For this review, take the finished solid that the model builds, in its own axes (mm). Coordinates: 2 decimals unless noted, no trailing zeros. Write each loop counter-clockwise with the first axis right and the second up, starting at its lowest first coordinate (ties: lowest second). Pieces come first, ordered by that corner, then holes. Notation, with made-up numbers: (2, 5.5) -> (21, 5.5) arc R23 cw to (21, 18.5) -> close; hole circle Ø7 at (77, -21). An arc over 180 degrees is marked (long way). Put each result on its own line as item: value. Start each with the question number.
Item 1: Consider section B-B on z = -168. Give the boundary of the cut face in (x, y) (3 decimals), and give its area (3 significant figures).
Item 2: Consider section A-A on y = 0.7. Give the boundary of the cut face in (x, z).
Item 3: Consider section C-C on x = 312.5. Give the boundary of the cut face in (y, z) (3 decimals).
Item 4: To check wall thickness, follow L1, parallel to Z at x = -130, y = 1.15; L2, parallel to X at y = 1.05, z = -150; L3, parallel to X at y = 2.15, z = -210. State the ranges of each line that lie inside material, in increasing order.
```python
from build123d import *

# Parameters (mm, degrees)
BOSS_EXTRUDE1_DEPTH = 3.175
CUT_EXTRUDE1_REACH  = 850.534


with BuildPart() as part:
    # Sketch1 → Boss-Extrude1 (new body)
    with BuildSketch(Plane(origin=(0, 0, 0), x_dir=(1, 0, 0), z_dir=(0, 1, 0))):
        with BuildLine():
            Line((-600, 0), (600, 0))
            ThreePointArc((600, 0), (0, 600), (-600, 0))
        make_face()
    extrude(amount=BOSS_EXTRUDE1_DEPTH)

    # Sketch2 → Cut-Extrude1 (cut, up to next)
    with BuildSketch(Plane(origin=(0, 3.175, 0), x_dir=(1, 0, 0), z_dir=(0, 1, 0)), mode=Mode.PRIVATE) as cut_extrude1_sk1:
        with BuildLine():
            Line((-130, 205), (-130, 210))
            Line((-130, 210), (-125, 210))
            ThreePointArc((-125, 210), (-133.535533906, 213.535533906), (-130, 205))
        make_face()
    cut_extrude1_tool1 = extrude(cut_extrude1_sk1.sketch, amount=-CUT_EXTRUDE1_REACH, mode=Mode.PRIVATE) & part.part
    # Sketch2 → Cut-Extrude1 (cut, up to next)
    with BuildSketch(Plane(origin=(0, 3.175, 0), x_dir=(1, 0, 0), z_dir=(0, 1, 0)), mode=Mode.PRIVATE) as cut_extrude1_sk2:
        with BuildLine():
            Line((-125, 210), (-130, 210))
            Line((-130, 210), (-130, 205))
            ThreePointArc((-130, 205), (-126.464466094, 206.464466094), (-125, 210))
        make_face()
    cut_extrude1_tool2 = extrude(cut_extrude1_sk2.sketch, amount=-CUT_EXTRUDE1_REACH, mode=Mode.PRIVATE) & part.part
    # Sketch2 → Cut-Extrude1 (cut, up to next)
    with BuildSketch(Plane(origin=(0, 3.175, 0), x_dir=(1, 0, 0), z_dir=(0, 1, 0)), mode=Mode.PRIVATE) as cut_extrude1_sk3:
        with BuildLine():
            Line((-130, 205), (-130, 210))
            Line((-130, 210), (-125, 210))
            ThreePointArc((-125, 210), (-133.535533906, 213.535533906), (-130, 205))
        make_face()
    cut_extrude1_tool3 = extrude(cut_extrude1_sk3.sketch, amount=-CUT_EXTRUDE1_REACH, mode=Mode.PRIVATE) & part.part
    # Sketch2 → Cut-Extrude1 (cut, up to next)
    with BuildSketch(Plane(origin=(0, 3.175, 0), x_dir=(1, 0, 0), z_dir=(0, 1, 0)), mode=Mode.PRIVATE) as cut_extrude1_sk4:
        with BuildLine():
            Line((-125, 210), (-130, 210))
            Line((-130, 210), (-130, 205))
            ThreePointArc((-130, 205), (-126.464466094, 206.464466094), (-125, 210))
        make_face()
    cut_extrude1_tool4 = extrude(cut_extrude1_sk4.sketch, amount=-CUT_EXTRUDE1_REACH, mode=Mode.PRIVATE) & part.part
    # Sketch2 → Cut-Extrude1 (cut, up to next)
    with BuildSketch(Plane(origin=(0, 3.175, 0), x_dir=(1, 0, 0), z_dir=(0, 1, 0)), mode=Mode.PRIVATE) as cut_extrude1_sk5:
        with BuildLine():
            ThreePointArc((-125, 150), (-126.464466094, 153.535533906), (-130, 155))
            Line((-130, 155), (-130, 150))
            Line((-130, 150), (-125, 150))
        make_face()
    cut_extrude1_tool5 = extrude(cut_extrude1_sk5.sketch, amount=-CUT_EXTRUDE1_REACH, mode=Mode.PRIVATE) & part.part
    # Sketch2 → Cut-Extrude1 (cut, up to next)
    with BuildSketch(Plane(origin=(0, 3.175, 0), x_dir=(1, 0, 0), z_dir=(0, 1, 0)), mode=Mode.PRIVATE) as cut_extrude1_sk6:
        with BuildLine():
            Line((-130, 150), (-130, 155))
            ThreePointArc((-130, 155), (-133.535533906, 146.464466094), (-125, 150))
            Line((-125, 150), (-130, 150))
        make_face()
    cut_extrude1_tool6 = extrude(cut_extrude1_sk6.sketch, amount=-CUT_EXTRUDE1_REACH, mode=Mode.PRIVATE) & part.part
    # Sketch2 → Cut-Extrude1 (cut, up to next)
    with BuildSketch(Plane(origin=(0, 3.175, 0), x_dir=(1, 0, 0), z_dir=(0, 1, 0)), mode=Mode.PRIVATE) as cut_extrude1_sk7:
        with BuildLine():
            ThreePointArc((-125, 150), (-126.464466094, 153.535533906), (-130, 155))
            Line((-130, 155), (-130, 150))
            Line((-130, 150), (-125, 150))
        make_face()
    cut_extrude1_tool7 = extrude(cut_extrude1_sk7.sketch, amount=-CUT_EXTRUDE1_REACH, mode=Mode.PRIVATE) & part.part
    # Sketch2 → Cut-Extrude1 (cut, up to next)
    with BuildSketch(Plane(origin=(0, 3.175, 0), x_dir=(1, 0, 0), z_dir=(0, 1, 0)), mode=Mode.PRIVATE) as cut_extrude1_sk8:
        with BuildLine():
            Line((-130, 150), (-130, 155))
            ThreePointArc((-130, 155), (-133.535533906, 146.464466094), (-125, 150))
            Line((-125, 150), (-130, 150))
        make_face()
    cut_extrude1_tool8 = extrude(cut_extrude1_sk8.sketch, amount=-CUT_EXTRUDE1_REACH, mode=Mode.PRIVATE) & part.part
    # Sketch2 → Cut-Extrude1 (cut, up to next)
    with BuildSketch(Plane(origin=(0, 3.175, 0), x_dir=(1, 0, 0), z_dir=(0, 1, 0)), mode=Mode.PRIVATE) as cut_extrude1_sk9:
        with BuildLine():
            ThreePointArc((135, 150), (133.535533906, 153.535533906), (130, 155))
            Line((130, 155), (130, 150))
            Line((130, 150), (125, 150))
            ThreePointArc((125, 150), (130, 145), (135, 150))
        make_face()
    cut_extrude1_tool9 = extrude(cut_extrude1_sk9.sketch, amount=-CUT_EXTRUDE1_REACH, mode=Mode.PRIVATE) & part.part
    # Sketch2 → Cut-Extrude1 (cut, up to next)
    with BuildSketch(Plane(origin=(0, 3.175, 0), x_dir=(1, 0, 0), z_dir=(0, 1, 0)), mode=Mode.PRIVATE) as cut_extrude1_sk10:
        with BuildLine():
            Line((130, 150), (130, 155))
            ThreePointArc((130, 155), (126.464466094, 153.535533906), (125, 150))
            Line((125, 150), (130, 150))
        make_face()
    cut_extrude1_tool10 = extrude(cut_extrude1_sk10.sketch, amount=-CUT_EXTRUDE1_REACH, mode=Mode.PRIVATE) & part.part
    # Sketch2 → Cut-Extrude1 (cut, up to next)
    with BuildSketch(Plane(origin=(0, 3.175, 0), x_dir=(1, 0, 0), z_dir=(0, 1, 0)), mode=Mode.PRIVATE) as cut_extrude1_sk11:
        with BuildLine():
            ThreePointArc((135, 150), (133.535533906, 153.535533906), (130, 155))
            Line((130, 155), (130, 150))
            Line((130, 150), (125, 150))
            ThreePointArc((125, 150), (130, 145), (135, 150))
        make_face()
    cut_extrude1_tool11 = extrude(cut_extrude1_sk11.sketch, amount=-CUT_EXTRUDE1_REACH, mode=Mode.PRIVATE) & part.part
    # Sketch2 → Cut-Extrude1 (cut, up to next)
    with BuildSketch(Plane(origin=(0, 3.175, 0), x_dir=(1, 0, 0), z_dir=(0, 1, 0)), mode=Mode.PRIVATE) as cut_extrude1_sk12:
        with BuildLine():
            Line((130, 150), (130, 155))
            ThreePointArc((130, 155), (126.464466094, 153.535533906), (125, 150))
            Line((125, 150), (130, 150))
        make_face()
    cut_extrude1_tool12 = extrude(cut_extrude1_sk12.sketch, amount=-CUT_EXTRUDE1_REACH, mode=Mode.PRIVATE) & part.part
    # Sketch2 → Cut-Extrude1 (cut, up to next)
    with BuildSketch(Plane(origin=(0, 3.175, 0), x_dir=(1, 0, 0), z_dir=(0, 1, 0)), mode=Mode.PRIVATE) as cut_extrude1_sk13:
        with BuildLine():
            ThreePointArc((135, 210), (130, 215), (125, 210))
            Line((125, 210), (130, 210))
            Line((130, 210), (130, 205))
            ThreePointArc((130, 205), (133.535533906, 206.464466094), (135, 210))
        make_face()
    cut_extrude1_tool13 = extrude(cut_extrude1_sk13.sketch, amount=-CUT_EXTRUDE1_REACH, mode=Mode.PRIVATE) & part.part
    # Sketch2 → Cut-Extrude1 (cut, up to next)
    with BuildSketch(Plane(origin=(0, 3.175, 0), x_dir=(1, 0, 0), z_dir=(0, 1, 0)), mode=Mode.PRIVATE) as cut_extrude1_sk14:
        with BuildLine():
            Line((130, 210), (125, 210))
            ThreePointArc((125, 210), (126.464466094, 206.464466094), (130, 205))
            Line((130, 205), (130, 210))
        make_face()
    cut_extrude1_tool14 = extrude(cut_extrude1_sk14.sketch, amount=-CUT_EXTRUDE1_REACH, mode=Mode.PRIVATE) & part.part
    # Sketch2 → Cut-Extrude1 (cut, up to next)
    with BuildSketch(Plane(origin=(0, 3.175, 0), x_dir=(1, 0, 0), z_dir=(0, 1, 0)), mode=Mode.PRIVATE) as cut_extrude1_sk15:
        with BuildLine():
            ThreePointArc((135, 210), (130, 215), (125, 210))
            Line((125, 210), (130, 210))
            Line((130, 210), (130, 205))
            ThreePointArc((130, 205), (133.535533906, 206.464466094), (135, 210))
        make_face()
    cut_extrude1_tool15 = extrude(cut_extrude1_sk15.sketch, amount=-CUT_EXTRUDE1_REACH, mode=Mode.PRIVATE) & part.part
    # Sketch2 → Cut-Extrude1 (cut, up to next)
    with BuildSketch(Plane(origin=(0, 3.175, 0), x_dir=(1, 0, 0), z_dir=(0, 1, 0)), mode=Mode.PRIVATE) as cut_extrude1_sk16:
        with BuildLine():
            Line((130, 210), (125, 210))
            ThreePointArc((125, 210), (126.464466094, 206.464466094), (130, 205))
            Line((130, 205), (130, 210))
        make_face()
    cut_extrude1_tool16 = extrude(cut_extrude1_sk16.sketch, amount=-CUT_EXTRUDE1_REACH, mode=Mode.PRIVATE) & part.part
    add(cut_extrude1_tool1.solids().sort_by_distance((-130.707355, 3.175, -210.707355))[0], mode=Mode.SUBTRACT)
    add(cut_extrude1_tool2.solids().sort_by_distance((-127.877934, 3.175, -207.877934))[0], mode=Mode.SUBTRACT)
    add(cut_extrude1_tool3.solids().sort_by_distance((-130.707355, 3.175, -210.707355))[0], mode=Mode.SUBTRACT)
    add(cut_extrude1_tool4.solids().sort_by_distance((-127.877934, 3.175, -207.877934))[0], mode=Mode.SUBTRACT)
    add(cut_extrude1_tool5.solids().sort_by_distance((-127.877934, 3.175, -152.122066))[0], mode=Mode.SUBTRACT)
    add(cut_extrude1_tool6.solids().sort_by_distance((-130.707355, 3.175, -149.292645))[0], mode=Mode.SUBTRACT)
    add(cut_extrude1_tool7.solids().sort_by_distance((-127.877934, 3.175, -152.122066))[0], mode=Mode.SUBTRACT)
    add(cut_extrude1_tool8.solids().sort_by_distance((-130.707355, 3.175, -149.292645))[0], mode=Mode.SUBTRACT)
    add(cut_extrude1_tool9.solids().sort_by_distance((130.707355, 3.175, -149.292645))[0], mode=Mode.SUBTRACT)
    add(cut_extrude1_tool10.solids().sort_by_distance((127.877934, 3.175, -152.122066))[0], mode=Mode.SUBTRACT)
    add(cut_extrude1_tool11.solids().sort_by_distance((130.707355, 3.175, -149.292645))[0], mode=Mode.SUBTRACT)
    add(cut_extrude1_tool12.solids().sort_by_distance((127.877934, 3.175, -152.122066))[0], mode=Mode.SUBTRACT)
    add(cut_extrude1_tool13.solids().sort_by_distance((130.707355, 3.175, -210.707355))[0], mode=Mode.SUBTRACT)
    add(cut_extrude1_tool14.solids().sort_by_distance((127.877934, 3.175, -207.877934))[0], mode=Mode.SUBTRACT)
    add(cut_extrude1_tool15.solids().sort_by_distance((130.707355, 3.175, -210.707355))[0], mode=Mode.SUBTRACT)
    add(cut_extrude1_tool16.solids().sort_by_distance((127.877934, 3.175, -207.877934))[0], mode=Mode.SUBTRACT)


solid = part.part
```
Return value:
1. outline: (-576, 0) -> (576, 0) -> (576, 3.175) -> (-576, 3.175) -> close
1. area: 3,660 mm^2
2. outline: (-600, 0) arc R600 ccw to (600, 0) -> close; hole circle Ø10 at (-130, -210); hole circle Ø10 at (-130, -150); hole circle Ø10 at (130, -210); hole circle Ø10 at (130, -150)
3. outline: (0, -512.195) -> (3.175, -512.195) -> (3.175, 0) -> (0, 0) -> close
4. L1: -585.75 to -215, -205 to -155, -145 to 0
4. L2: -580.95 to -135, -125 to 125, 135 to 580.95
4. L3: -562.05 to -135, -125 to 125, 135 to 562.05
